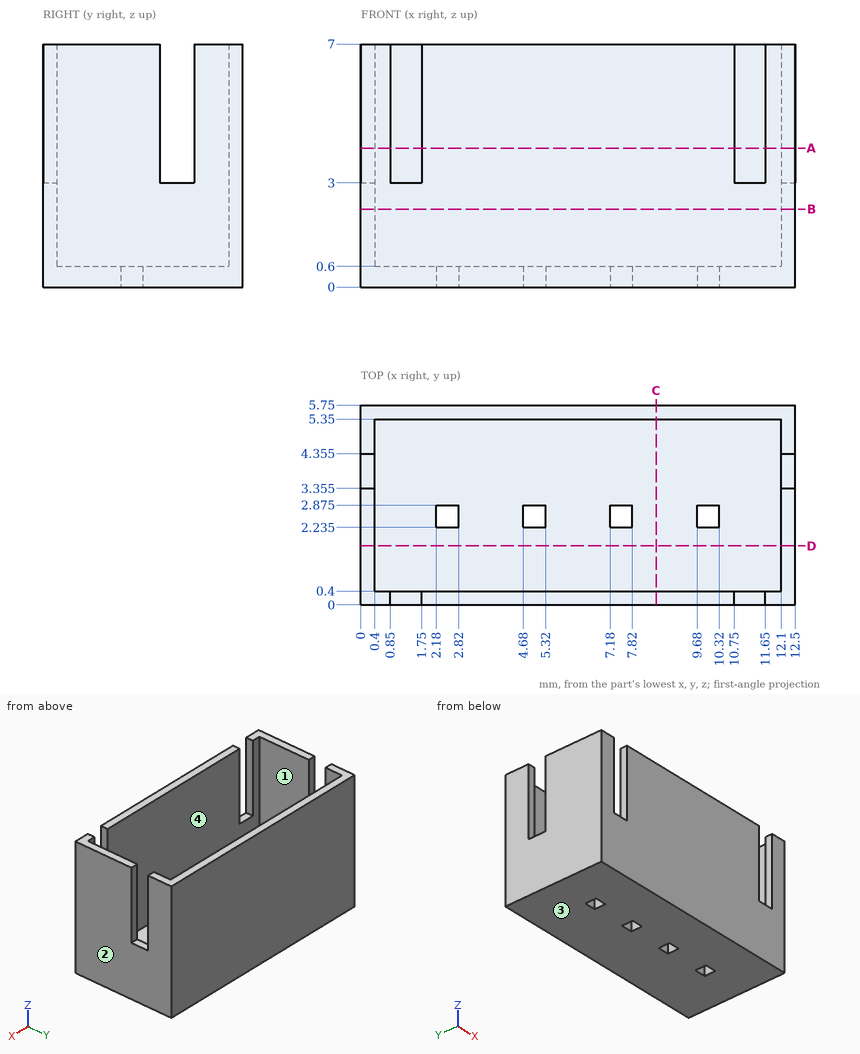
Input: dimensioned drawing with shaded views. Units: mm. Origin: part minimum x, y, z. Coordinates: 2 decimals unless noted, no trailing zeros. Loops run counter-clockwise (first coordinate to the right, second up) from the corner with the lowest first, then second, coordinate; pieces in that order, holes last. Notation, with made-up numbers: M -26,1 L -21,1 A19 cw -21,22 Z; hole C 48,32.25 d6. An arc over 180 degrees is marked long. Use a Markdown table: item, result. Add a question column.
Q1. Section query D-D, the plane y = 1.7. Return loops of the section in (x, z), and give its area (3 significant figures).
Q2. Draft query along X for the marked faces 1, 2, 3 and 4. Return one class per face: pulls with the +X half, pulls with the -X half, needs draft (parallel to the pull), parting line crosses it, or undercut.
Q3. Material intervals for L1, parallel to Y at x = 1.25, z = 1.5; L2, parallel to X at y = 5.05, z = 5.25; L3, parallel to Z at x = 2.5, y = 3.6, sorted ascending.
Q4. Section query B-B, the plane z = 2.25. Return loops of the section in (x, y).
Q5. Section query C-C, the plane x = 8.5. Return loops of the section in (y, z), and give its area (3 significant figures).
Q6. Section query A-A, the plane z = 4. Return loops of the section in (x, y) (3 decimals), and give its area (3 significant figures).
Result:
| question | item | result |
|---|---|---|
| 1 | outline | M 0,0 L 12.5,0 L 12.5,7 L 12.1,7 L 12.1,0.6 L 0.4,0.6 L 0.4,7 L 0,7 Z |
| 1 | area | 12.6 mm2 |
| 2 | face 1 | undercut |
| 2 | face 2 | pulls with the +X half |
| 2 | face 3 | needs draft |
| 2 | face 4 | undercut |
| 3 | L1 | y = 0 to 0.4, 5.35 to 5.75 |
| 3 | L2 | x = 0 to 0.4, 12.1 to 12.5 |
| 3 | L3 | z = 0 to 0.6 |
| 4 | outline | M 0,0 L 12.5,0 L 12.5,5.75 L 0,5.75 Z; hole M 0.4,0.4 L 12.1,0.4 L 12.1,5.35 L 0.4,5.35 Z |
| 5 | outline | M 0,0 L 5.75,0 L 5.75,7 L 5.35,7 L 5.35,0.6 L 0.4,0.6 L 0.4,7 L 0,7 Z |
| 5 | area | 8.57 mm2 |
| 6 | outline | M 0,0 L 0.85,0 L 0.85,0.4 L 0.4,0.4 L 0.4,3.355 L 0,3.355 Z; M 0,4.355 L 0.4,4.355 L 0.4,5.35 L 12.1,5.35 L 12.1,4.355 L 12.5,4.355 L 12.5,5.75 L 0,5.75 Z; M 1.75,0 L 10.75,0 L 10.75,0.4 L 1.75,0.4 Z; M 11.65,0 L 12.5,0 L 12.5,3.355 L 12.1,3.355 L 12.1,0.4 L 11.65,0.4 Z |
| 6 | area | 12.4 mm2 |
